Verification items for this drawing (mm, ordinates from the low corner). Coordinates: 2 decimals unless noted, no trailing zeros.
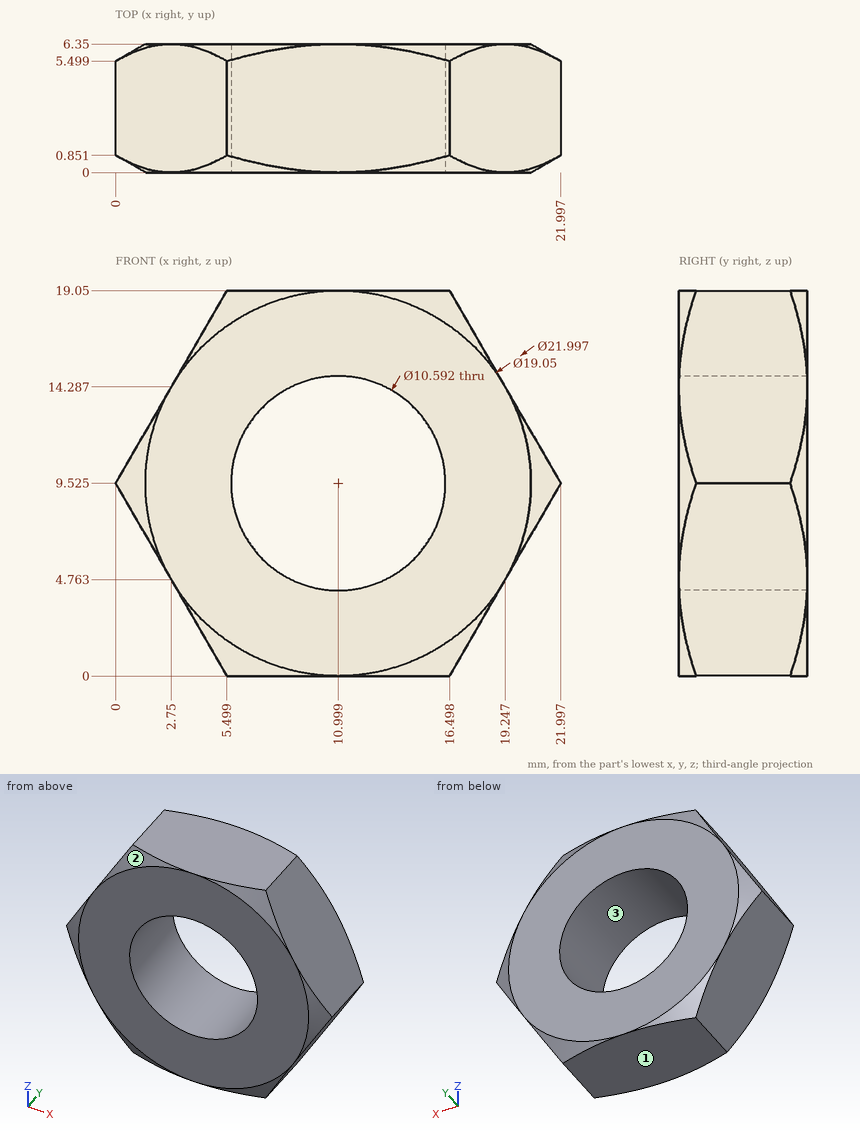
(1) Gauge pin test, flat ends, axial feed: P1, Ø3, axis at y = 2.5, z = 3, coming from the -X side; P2, Ø2, axis at x = 3, y = 1, coming from the +Z side (1 decimal); P3, Ø3, axis at y = 4.5, z = 16.5, coming from the -X side. Record the tip position at first contact, or that the pin passes through.
(2) Scan lines: line 1 along X through (y, z) = (2.75, 12.5) (1 decimal); line 2 along X through (y, z) = (3.25, 7) (1 decimal); line 3 along Z through (x, y) = (11.75, 3). Record each from-to range of solid material in increasing order.
(3) Draft check along X on the marked faces 1, 2 and 3. Enter one of: pulls with the +X half, pulls with the -X half, needs draft (parallel to the pull), parting line crosses it, or undercut.
Determined:
1. P1: stops at x = 2.9
1. P2: stops at z = 16.5
1. P3: stops at x = 3.16
2. line 1: x = 1.7 to 6.6, 15.4 to 20.3
2. line 2: x = 1.5 to 6.3, 15.7 to 20.5
2. line 3: z = 0 to 4.28, 14.77 to 19.05
3. face 1: needs draft
3. face 2: pulls with the -X half
3. face 3: undercut
